Could you check a few things on this model? Use its own coordinates, in mm. Give positions to 0.01 mm unless a question says otherwise; leave off trailing zeros. Loops run counter-clockwise (first coordinate to the right, second up) from the corner with the lowest first, then second, coordinate; pieces in that order, holes last. Notation, with made-up numbers: (16, 57) -> (59, 57) arc R9 ccw to (59, 62) -> close; hole circle Ø3 at (-0.75, 49.25). An arc over 180 degrees is marked (long way). Write each question's results on one line, items separated by ' | '. Start each with the question number.
Q1. If I drill on line 1 along Y through (x, z) = (110, 2); line 2 along Y through (x, z) = (-79, 16.5); line 3 along X through (y, z) = (93, 18), over which ranges is the centre line in solid material (lowest first)?
Q2. If we section it at C-C, the plane z = 9.5: List the corners of the cut face in (x, y) for me, plus the area to 3 significant figures.
Q3. Will these pins go through, and if not, where does the flat tip stop? P1, Ø4, axis at y = 61.5, z = 11.5, coming from the -X side; P2, Ø4, axis at x = 90.5, y = 121.5, coming from the -Z side; P3, Ø6, axis at x = -10, z = 16.5, coming from the +Y side; P4, Ø1, axis at y = -113, z = 4, coming from the +X side.
Autodesk Inventor part; units mm, degrees
ref_plane "YZ Plane" through (0, 0, 0) normal (1, 0, 0) x (0, 1, 0)
ref_plane "XZ Plane" through (0, 0, 0) normal (0, 1, 0) x (-1, 0, 0)
ref_plane "XY Plane" through (0, 0, 0) normal (0, 0, 1) x (1, 0, 0)
sketch "Skizze1" plane through (0, 0, 0) normal (0, 0, 1) x (1, 0, 0)
  line L0 (0, -315) -> (0, 315)
  line L1 (-350, 0) -> (350, 0)
  line L2 (-250, 225) -> (250, 225)
  line L3 (250, 225) -> (250, -225)
  line L4 (250, -225) -> (-250, -225)
  line L5 (-250, -225) -> (-250, 225)
  point P0 (0, 0)
  dimension "d0" = 500
  dimension "d1" = 450
extrude "Extrusion1" add sketch "Skizze1" along normal blind 20
chamfer "Fase1" distance 20 angle 45 4 edges at (-250, 0, 0) (0, 225, 0) (250, 0, 0) (0, -225, 0)
properties part number "Wand1"
Final values:
1) line 1: y = -207 to 207 | line 2: y = -221.5 to 221.5 | line 3: x = -248 to 248
2) outline: (-239.5, -214.5) -> (239.5, -214.5) -> (239.5, 214.5) -> (-239.5, 214.5) -> close | area: 205,000 mm²
3) P1: stops at x = -243.5 | P2: stops at z = 0 | P3: stops at y = 224.5 | P4: stops at x = 234.5
